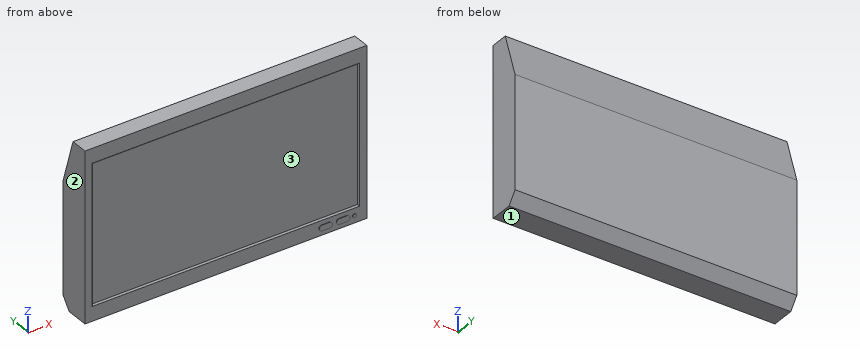
```python
from build123d import *

# Parameters (mm, degrees)
F1_DEPTH     = 317.5
F2_W         = 606.8687809474
F2_H         = 319.4243614871
F3_DEPTH     = 3.175
F4_T4_DEPTH  = 345.5526606448
F4_T9_DEPTH  = 632.9970801051
F4_T14_DEPTH = 345.5526606448
F4_T19_DEPTH = 632.9970801051
F5_R         = 4.2314330569
F6_DEPTH     = 1.27


# Not quite as in the source:
# - a fillet or chamfer that OpenCascade refuses, or shapes differently, is made with other operations: its cross-section is extruded or revolved along the edge and cut away or added


with BuildPart() as f1:
    # F0 (on Right) → F1 (new body, symmetric)
    with BuildSketch(Plane.YZ):
        Polygon((0, 381), (0, 0), (51.4319166541, 0), (71.12, 25.4), (71.12, 279.4), (39.1150377691, 381), align=None)
    extrude(amount=F1_DEPTH, both=True)

    # F2 (on face) → F3 (cut)
    with BuildSketch(Plane.XZ):
        with Locations((0, 190.5)):
            Rectangle(F2_W, F2_H)
    extrude(amount=-F3_DEPTH, mode=Mode.SUBTRACT)

    # F4: chamfer of 5.08 on 4 edges, made by hand


with BuildPart() as f4_tool2:
    # F4_s3 → F4_t4 (new body)
    with BuildSketch(Plane.XY.offset(363.2763303224)):
        Polygon((-303.4343904737, -1.905), (-298.3543904737, 3.175), (-303.4343904737, 3.175), align=None)
    extrude(amount=-F4_T4_DEPTH)

    split(bisect_by=Plane.XZ, keep=Keep.BOTTOM)


with BuildPart() as f1_1:
    add(f1.part)

    # F4_t1: union F4_tool2
    add(f4_tool2.part)


with BuildPart() as f4_tool7:
    # F4_s8 → F4_t9 (new body)
    with BuildSketch(Plane.YZ.offset(316.4985400526)):
        Polygon((-1.905, 350.2121807435), (3.175, 345.1321807435), (3.175, 350.2121807435), align=None)
    extrude(amount=-F4_T9_DEPTH)

    split(bisect_by=Plane.XZ, keep=Keep.BOTTOM)


with BuildPart() as f1_2:
    add(f1_1.part)

    # F4_t6: union F4_tool7
    add(f4_tool7.part)


with BuildPart() as f4_tool12:
    # F4_s13 → F4_t14 (new body)
    with BuildSketch(Plane.XY.offset(17.7236696776)):
        Polygon((303.4343904737, -1.905), (298.3543904737, 3.175), (303.4343904737, 3.175), align=None)
    extrude(amount=F4_T14_DEPTH)

    split(bisect_by=Plane.XZ, keep=Keep.BOTTOM)


with BuildPart() as f1_3:
    add(f1_2.part)

    # F4_t11: union F4_tool12
    add(f4_tool12.part)


with BuildPart() as f4_tool17:
    # F4_s18 → F4_t19 (new body)
    with BuildSketch(Plane.YZ.offset(-316.4985400526)):
        Polygon((-1.905, 30.7878192565), (3.175, 35.8678192565), (3.175, 30.7878192565), align=None)
    extrude(amount=F4_T19_DEPTH)

    split(bisect_by=Plane.XZ, keep=Keep.BOTTOM)


with BuildPart() as f1_4:
    add(f1_3.part)

    # F4_t16: union F4_tool17
    add(f4_tool17.part)

    # F5 (on face) → F6 (join)
    with BuildSketch(Plane.XZ):
        with BuildLine():
            ThreePointArc((233.1511284661, 10.1901956652), (239.5011284661, 16.5401956652), (233.1511284661, 22.8901956652))
            Line((233.1511284661, 22.8901956652), (215.7576586556, 22.8901956652))
            ThreePointArc((215.7576586556, 22.8901956652), (209.4076586556, 16.5401956652), (215.7576586556, 10.1901956652))
            Line((215.7576586556, 10.1901956652), (233.1511284661, 10.1901956652))
        make_face()
        with BuildLine():
            ThreePointArc((272.4028527737, 10.1901956652), (278.7528527737, 16.5401956652), (272.4028527737, 22.8901956652))
            Line((272.4028527737, 22.8901956652), (255.0093829632, 22.8901956652))
            ThreePointArc((255.0093829632, 22.8901956652), (248.6593829632, 16.5401956652), (255.0093829632, 10.1901956652))
            Line((255.0093829632, 10.1901956652), (272.4028527737, 10.1901956652))
        make_face()
        with Locations((289.2993986607, 16.5401956652)):
            Circle(F5_R)
    extrude(amount=F6_DEPTH)


solid = f1_4.part
```
Verification items for the finished model (mm, model axes). Face numbers are marked on the shaded views. Coordinates: 2 decimals unless noted, no trailing zeros. Write each loop counter-clockwise with the first axis right and the second up, starting at its lowest first coordinate (ties: lowest second). Pieces come first, ordered by that corner, then holes. Notation, with made-up numbers: (-28.75, 3.5) - (-1.75, 3.5) arc R31 cw to (-1.75, 31.5) - close; hole circle Ø2 at (-30, 28.5). An arc over 180 degrees is marked (long way). Write item = value, one per line.
Q1. Material ranges on L1, parallel to Z at x = 201, y = 2; L2, parallel to Z at x = -78, y = 3; L3, parallel to Y at x = 73.5, z = 148 (3 decimals), recorded low to high. Write a range as from..to.
Answer:
L1 = 0..34.69, 346.31..381
L2 = 0..35.69, 345.31..381
L3 = 3.175..71.12
Q2. Cross-section at B-B (z = 63.5). Enter the section's corners in (x, y) (3 decimals).
Answer:
outline = (-317.5, 0) - (-301.529, 0) - (-298.354, 3.175) - (298.354, 3.175) - (301.529, 0) - (317.5, 0) - (317.5, 71.12) - (-317.5, 71.12) - close
Q3. Cross-section at D-D (z = 307). Enter the section's corners in (x, y) (3 decimals).
Answer:
outline = (-317.5, 0) - (-301.529, 0) - (-298.354, 3.175) - (298.354, 3.175) - (301.529, 0) - (317.5, 0) - (317.5, 62.426) - (-317.5, 62.426) - close
Q4. Go/stop test with flat-tipped pins: pin 1 Ø1 at (x, y) = (268, -1) entering from -Z; pin 2 Ø5 at (x, y) = (209.5, 8.5) entering from -Z; pin 3 Ø12 at (x, y) = (123.5, 58) entering from -Z; pin 4 Ø4 at (x, y) = (-88.5, 62) entering from -Z. Record where each tip stops, or that it passes through.
Answer:
pin_1 = 10.19
pin_2 = 0
pin_3 = 0.73
pin_4 = 11.05
Q5. Cross-section at A-A (x = -127.5). Enter the section's corners in (y, z) (3 decimals), plus the area to 3 significant figures.
Answer:
outline = (0, 0) - (51.432, 0) - (71.12, 25.4) - (71.12, 279.4) - (39.115, 381) - (0, 381) - (0, 348.307) - (3.175, 345.132) - (3.175, 35.868) - (0, 32.693) - close
area = 24,200 mm²
Q6. Mould release check, pull along X, two halves, no side actions. Record for the marked faces 1, 2 and 3: released by +X, released by -X, zero draft, split by the parting line, or undercut.
Answer:
face_1 = zero draft
face_2 = released by -X
face_3 = undercut
Q7. Cross-section at C-C (y = 58). Enter the section's corners in (x, z), plus the area to 3 significant figures.
Answer:
outline = (-317.5, 8.47) - (317.5, 8.47) - (317.5, 321.05) - (-317.5, 321.05) - close
area = 198,000 mm²
